Geometry check sheet. Reference: the model listing, model coordinates, mm. A direction names the side the tool comes from. Coordinates: 2 decimals unless noted, no trailing zeros. Order: outer loops, then holes, each group sorted by start corner. A loop starts at its lowest first (then second) coordinate and runs counter-clockwise, first axis right, second up. Notation, with made-up numbers: (76.25, 89.25) - (101.25, 89.25) arc R15 cw to (101.25, 117.25) - close; hole circle Ø6 at (74.5, -5). An arc over 180 degrees is marked (long way). Return JSON: item names as keys, results as strings. Group by question number.
Item 1: Section check B-B on z = 40. Enter the section's corners in (x, y).
Item 2: Section check D-D on x = 0. Enter the section's corners in (y, z), then the cut area to 3 significant figures.
Item 3: Gauge pin test, flat ends, axial feed: pin 1 (6 mm diameter, centred on y = 13.5, z = -5.5, fed in from -X); pin 2 (9 mm diameter, centred on x = 3.5, y = 11, fed in from +Z); pin 3 (14.5 mm diameter, centred on x = -3.5, y = 9, fed in from -Z). Record the tip position at first contact, or that the pin passes through.
Item 4: Section check A-A on x = 40. Enter the section's corners in (y, z), then the cut area to 3 significant figures.
Item 5: Scan lines: probe 1 along Z at (x, y) = (-40, -8.75); probe 2 along Z at (x, y) = (6.5, 8.75). Record each from-to range of solid material in increasing order.
Item 6: Tool access check on faces 1 (the flat face through (35, 9, 0)), 2 (the flat face through (13, 0, 0)), 3 (the cylindrical face through (30.72, 8.87, -30.49)). Record the directions out of +Z, -Z, +X, -X, +Y, -Y that give a thin tool (end or side, any length) a straight path to the whole face; none if there is none.
Item 7: Section check C-C on y = -8.25. Enter the section's corners in (x, z).
from build123d import *

# Parameters (mm, degrees)
F0_W     = 100
F0_H     = 100
F0_R     = 4
F0_R_2   = 10
F1_DEPTH = 12
F3_DEPTH = 18


with BuildPart() as f1:
    # F0 (on Front) → F1 (new body)
    with BuildSketch(Plane.XZ):
        Rectangle(F0_W, F0_H)
        with Locations((-40, -40)):
            Circle(F0_R, mode=Mode.SUBTRACT)
        with Locations((40, -40)):
            Circle(F0_R, mode=Mode.SUBTRACT)
        with Locations((-40, 40)):
            Circle(F0_R, mode=Mode.SUBTRACT)
        Circle(F0_R_2, mode=Mode.SUBTRACT)
        with Locations((40, 40)):
            Circle(F0_R, mode=Mode.SUBTRACT)
    extrude(amount=F1_DEPTH)

    # F2 (on face) → F3 (join)
    with BuildSketch(Plane(origin=(0, 0, 0), x_dir=(-1, 0, 0), z_dir=(0, 1, 0))):
        with BuildLine():
            ThreePointArc((-20, 35), (-30.606602, 30.606602), (-35, 20))
            Line((-35, 20), (-35, -20))
            ThreePointArc((-35, -20), (-30.606602, -30.606602), (-20, -35))
            Line((-20, -35), (20, -35))
            ThreePointArc((20, -35), (30.606602, -30.606602), (35, -20))
            Line((35, -20), (35, 20))
            ThreePointArc((35, 20), (30.606602, 30.606602), (20, 35))
            Line((20, 35), (-20, 35))
        make_face()
        with BuildLine():
            Line((-30, -20), (-30, 20))
            ThreePointArc((-30, 20), (-27.071068, 27.071068), (-20, 30))
            Line((-20, 30), (20, 30))
            ThreePointArc((20, 30), (27.071068, 27.071068), (30, 20))
            Line((30, 20), (30, -20))
            ThreePointArc((30, -20), (27.071068, -27.071068), (20, -30))
            Line((20, -30), (-20, -30))
            ThreePointArc((-20, -30), (-27.071068, -27.071068), (-30, -20))
        make_face(mode=Mode.SUBTRACT)
    extrude(amount=F3_DEPTH)


solid = f1.part
Computed:
{
 "1": {"outline": "(-50, -12) - (-44, -12) - (-44, 0) - (-50, 0) - close; (-36, -12) - (36, -12) - (36, 0) - (-36, 0) - close; (44, -12) - (50, -12) - (50, 0) - (44, 0) - close"},
 "2": {"outline": "(-12, -50) - (0, -50) - (0, -35) - (18, -35) - (18, -30) - (0, -30) - (0, -10) - (-12, -10) - close; (-12, 10) - (0, 10) - (0, 30) - (18, 30) - (18, 35) - (0, 35) - (0, 50) - (-12, 50) - close", "area": "1,140 mm²"},
 "3": {"pin 1": "stops at x = -35", "pin 2": "stops at z = 35", "pin 3": "stops at z = -35"},
 "4": {"outline": "(-12, -50) - (0, -50) - (0, -44) - (-12, -44) - close; (-12, -36) - (0, -36) - (0, 36) - (-12, 36) - close; (-12, 44) - (0, 44) - (0, 50) - (-12, 50) - close", "area": "1,010 mm²"},
 "5": {"probe 1": "z = -50 to -44, -36 to 36, 44 to 50", "probe 2": "z = -35 to -30, 30 to 35"},
 "6": {"face 1": "+Z, -Z, +X, +Y", "face 2": "+Y", "face 3": "-Z, +X, +Y"},
 "7": {"outline": "(-50, -50) - (50, -50) - (50, 50) - (-50, 50) - close; hole circle Ø8 at (-40, -40); hole circle Ø8 at (-40, 40); hole circle Ø20 at (0, 0); hole circle Ø8 at (40, -40); hole circle Ø8 at (40, 40)"}
}
